from build123d import *

# Parameters (mm, degrees)
IZIM1_R                     = 22.86
Y_KSEKLIK_EKSTR_ZYON1_DEPTH = 44.45
IZIM2_R                     = 3.175
Y_KSEKLIK_EKSTR_ZYON2_DEPTH = 25.4
KES_EKSTR_ZYON1_DEPTH       = 7.62
RADYUS1_R                   = 1.524


with BuildPart() as part:
    # Çizim1 → Yükseklik-Ekstrüzyon1 (new body)
    with BuildSketch(Plane.XY):
        Circle(IZIM1_R)
    extrude(amount=Y_KSEKLIK_EKSTR_ZYON1_DEPTH)

    # Çizim2 → Yükseklik-Ekstrüzyon2 (add)
    with BuildSketch(Plane.XY.offset(44.45)):
        Circle(IZIM2_R)
    extrude(amount=Y_KSEKLIK_EKSTR_ZYON2_DEPTH)

    # Çizim3 → Kes-Ekstrüzyon1 (cut)
    with BuildSketch(Plane.XY.offset(44.45)):
        with BuildLine():
            Line((12.7, 0), (15.24, 0))
            ThreePointArc((15.24, 0), (13.198227154, 7.62), (7.62, 13.198227154))
            Line((7.62, 13.198227154), (6.35, 10.998522628))
            ThreePointArc((6.35, 10.998522628), (10.998522628, 6.35), (12.7, 0))
        make_face()
        with BuildLine():
            Line((8.89, 15.397931679), (10.16, 17.597636205))
            ThreePointArc((10.16, 17.597636205), (17.597636205, 10.16), (20.32, 0))
            Line((20.32, 0), (17.78, 0))
            ThreePointArc((17.78, 0), (15.397931679, 8.89), (8.89, 15.397931679))
        make_face()
        with BuildLine():
            Line((10.998522628, -6.35), (13.198227154, -7.62))
            ThreePointArc((13.198227154, -7.62), (7.62, -13.198227154), (0, -15.24))
            Line((0, -15.24), (0, -12.7))
            ThreePointArc((0, -12.7), (6.35, -10.998522628), (10.998522628, -6.35))
        make_face()
        with BuildLine():
            Line((0, -17.78), (0, -20.32))
            ThreePointArc((0, -20.32), (10.16, -17.597636205), (17.597636205, -10.16))
            Line((17.597636205, -10.16), (15.397931679, -8.89))
            ThreePointArc((15.397931679, -8.89), (8.89, -15.397931679), (0, -17.78))
        make_face()
        with BuildLine():
            Line((-6.35, -10.998522628), (-7.62, -13.198227154))
            ThreePointArc((-7.62, -13.198227154), (-13.198227154, -7.62), (-15.24, 0))
            Line((-15.24, 0), (-12.7, 0))
            ThreePointArc((-12.7, 0), (-10.998522628, -6.35), (-6.35, -10.998522628))
        make_face()
        with BuildLine():
            Line((-17.78, 0), (-20.32, 0))
            ThreePointArc((-20.32, 0), (-17.597636205, -10.16), (-10.16, -17.597636205))
            Line((-10.16, -17.597636205), (-8.89, -15.397931679))
            ThreePointArc((-8.89, -15.397931679), (-15.397931679, -8.89), (-17.78, 0))
        make_face()
        with BuildLine():
            Line((-10.998522628, 6.35), (-13.198227154, 7.62))
            ThreePointArc((-13.198227154, 7.62), (-7.62, 13.198227154), (0, 15.24))
            Line((0, 15.24), (0, 12.7))
            ThreePointArc((0, 12.7), (-6.35, 10.998522628), (-10.998522628, 6.35))
        make_face()
        with BuildLine():
            Line((0, 17.78), (0, 20.32))
            ThreePointArc((0, 20.32), (-10.16, 17.597636205), (-17.597636205, 10.16))
            Line((-17.597636205, 10.16), (-15.397931679, 8.89))
            ThreePointArc((-15.397931679, 8.89), (-8.89, 15.397931679), (0, 17.78))
        make_face()
    extrude(amount=-KES_EKSTR_ZYON1_DEPTH, mode=Mode.SUBTRACT)

    # Radyus1
    radyus1_edges = [part.edges().sort_by_distance(p)[0] for p in [
        (-22.86, 0, 44.45),
    ]]
    fillet(radyus1_edges, radius=RADYUS1_R)


solid = part.part
Part model, mm, in its own coordinate system. Give positions to 0.01 mm unless a question says otherwise; leave off trailing zeros. Order: outer loops, then holes, each group sorted by start corner. A loop starts at its lowest first (then second) coordinate and runs counter-clockwise, first axis right, second up. Notation, with made-up numbers: (-12.5, 74) - (-2.5, 74) arc R28 cw to (-2.5, 101) - close; hole circle Ø7 at (-26, 10.25). An arc over 180 degrees is marked (long way). One line per question, with ' | ' between items.
1. Band-saw the part on A-A on z = 17. List the corners of the cut face in (x, y), then the cut area to 3 significant figures.
Filled in:
outline: circle Ø45.72 at (0, 0) | area: 1,640 mm²
2. Drop flat-ended pins along their axis: P1, Ø3.5, axis at x = 15, y = 8.5, coming from the +Z side; P2, Ø2, axis at x = -14.5, z = 40, coming from the -Y side; P3, Ø1.3, axis at y = -14, z = 41, coming from the +X side. Give the stop position or say it passes through.
Filled in:
P1: z = 44.45 | P2: y = -18.45 | P3: x = 18.56
3. Drill centre lines: probe 1 along Y at (x, z) = (-5.5, 37.5); probe 2 along Z at (x, y) = (15, 7.5); probe 3 along Z at (x, y) = (-10, -17). Where is each one in solid material? Low to high.
Filled in:
probe 1: -22.19 to 11.45, 14.21 to 16.91, 19.56 to 22.19 | probe 2: 0 to 44.45 | probe 3: 0 to 36.83
4. Pull direction X, two halves, no side cores. Call faces 1 (the face through (14, 0, 41)), 2 (the face through (21.804, 6.867, 21.163)): +X half, -X half, draft (parallel to the pull), parting line (faces both ways), or undercut.
Filled in:
face 1: undercut | face 2: parting line
5. Band-saw the part on B-B on z = 60.5. List the corners of the cut face in (x, y) (3 decimals).
Filled in:
outline: circle Ø6.35 at (0, 0)
